The listing builds one solid part. Answer for the finished solid, in the listing's coordinates (mm). Round coordinates to 2 decimals unless told otherwise and drop trailing zeros. Write each loop counter-clockwise with the first axis right and the second up, starting at its lowest first coordinate (ties: lowest second). Pieces come first, ordered by that corner, then holes. Notation, with made-up numbers: M 72,5.5 L 79,5.5 A23 ccw 79,15.5 Z; hole C 52,25 d3. An arc over 180 degrees is marked long. One line per item, written item: value. Start each with the question number.
(1) Section A-A (z = 4.25) is taken. Determine the outline of the cut face in (x, y), plus the area to 3 significant figures.
(2) Section B-B (y = 14.5) is taken. Determine the outline of the cut face in (x, z).
(3) Section C-C (x = -5.8) is taken. Determine the outline of the cut face in (y, z), plus the area to 3 significant figures.
(4) Section D-D (z = 6.5) is taken. Determine the outline of the cut face in (x, y), plus the area to 3 significant figures.
(5) Consider probe 1 along Y at (x, z) = (-5.8, 2.75); probe 2 along Y at (x, z) = (-5.85, 4.75); probe 3 along Z at (x, y) = (-5.45, 16.25). Determine where each line is inside the solid, lowest interval first.
```python
from build123d import *

# Parameters (mm, degrees)
BOX001_W     = 2.71
BOX001_H     = 11
BOX001_DEPTH = 7.5
POCKET_DEPTH = 5
FILLET001_R  = 1


with BuildPart() as part:
    # Box001 → Box001 (new body)
    with BuildSketch(Plane(origin=(-7.36, 9.35, 0), x_dir=(1, 0, 0), z_dir=(0, 0, 1))):
        with Locations((1.355, 5.5)):
            Rectangle(BOX001_W, BOX001_H)
    extrude(amount=BOX001_DEPTH)

    # Sketch → Pocket (cut)
    with BuildSketch(Plane(origin=(-7.36, 9.35, 0), x_dir=(0, -1, 0), z_dir=(-1, 0, 0))):
        Polygon((-9.540607, 7.550952), (0.165381, -0.144127), (0.165381, 8.596624), align=None)
    extrude(amount=-POCKET_DEPTH, mode=Mode.SUBTRACT)

    # Fillet001
    fillet001_edges = [part.edges().sort_by_distance(p)[0] for p in [
        (-7.36, 20.35, 3.75),
        (-4.65, 20.35, 3.75),
    ]]
    fillet(fillet001_edges, radius=FILLET001_R)


solid = part.part
```
Recorded:
1. outline: M -7.36,14.73 L -4.65,14.73 L -4.65,19.35 A1 ccw -5.65,20.35 L -6.36,20.35 A1 ccw -7.36,19.35 Z
1. area: 14.8 mm2
2. outline: M -7.36,0 L -4.65,0 L -4.65,4.07 L -7.36,4.07 Z
3. outline: M 9.37,0 L 20.35,0 L 20.35,7.5 L 18.83,7.5 Z
3. area: 46.9 mm2
4. outline: M -7.36,17.57 L -4.65,17.57 L -4.65,19.35 A1 ccw -5.65,20.35 L -6.36,20.35 A1 ccw -7.36,19.35 Z
4. area: 7.12 mm2
5. probe 1: y = 12.84 to 20.35
5. probe 2: y = 15.36 to 20.35
5. probe 3: z = 0 to 5.46
